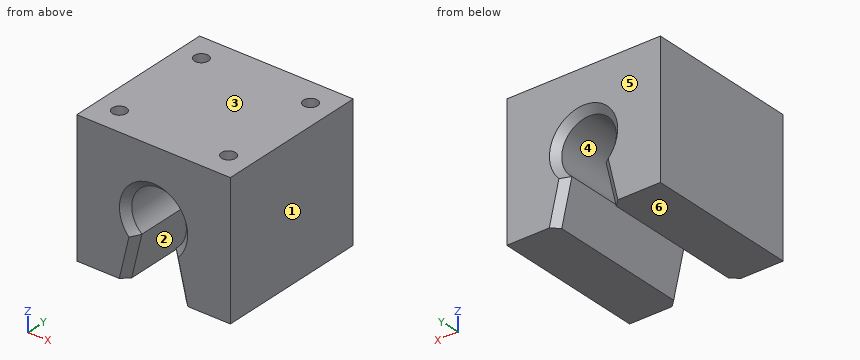
Autodesk Inventor part; units mm, degrees
ref_plane "YZ Plane" through (0, 0, 0) normal (1, 0, 0) x (0, 1, 0)
ref_plane "XZ Plane" through (0, 0, 0) normal (0, 1, 0) x (-1, 0, 0)
ref_plane "XY Plane" through (0, 0, 0) normal (0, 0, 1) x (1, 0, 0)
sketch "Skizze1" plane through (0, 0, 0) normal (0, 0, 1) x (1, 0, 0)
  line L0 (-22.5, -22.5) -> (22.5, -22.5)
  line L1 (22.5, -22.5) -> (22.5, 22.5)
  line L2 (22.5, 22.5) -> (-22.5, 22.5)
  line L3 (-22.5, 22.5) -> (-22.5, -22.5)
  line L4 (-22.5, -22.5) -> (22.5, 22.5) construction
  line L5 (22.5, -22.5) -> (-22.5, 22.5) construction
  point P0 (0, 0)
  dimension "d0" = 45
  dimension "d1" = 45
extrude "Extrusion1" add sketch "Skizze1" along normal blind 39
sketch "Skizze2" plane through (-22.5, -22.5, 0) normal (0, -1, 0) x (1, 0, 0)
  line L0 (0, 0) -> (45, 0)
  line L1 (45, 0) -> (45, 39)
  line L2 (0, 39) -> (45, 39)
  line L3 (0, 0) -> (0, 39)
  circle A0 centre (22.5, 19) radius 8
  line L4 (22.5, 0) -> (22.5, 39)
  line L5 (22.5, 19) -> (22.5, -6)
  line L6 (17.5, 12.755) -> (14.5, 0)
  line L7 (27.5, 12.755) -> (30.5, 0)
  dimension "d4" = 16
  dimension "d5" = 25
  dimension "d6" = 45
  dimension "d7" = 10
  dimension "d8" = 16
extrude "Extrusion2" cut sketch "Skizze2" against normal through all contours L6 A0 L4 L0 | L4 A0 L7 L0 | A0 L4 | L4 A0
chamfer "Fase1" distance 2 angle 45 6 edges at (0, -22.5, 27) (-6.5, -22.5, 6.3775) (6.5, -22.5, 6.3775) (0, 22.5, 27) (-6.5, 22.5, 6.3775) (6.5, 22.5, 6.3775)
ref_plane "Arbeitsebene1" through (-22.5, 0, 39) normal (0, 1, 0) x (1, 0, 0)
sketch "Skizze3" plane through (0, 0, 39) normal (0, 0, 1) x (1, 0, 0)
  line L0 (-22.5, -22.5) -> (22.5, -22.5)
  line L1 (22.5, -22.5) -> (22.5, 22.5)
  line L2 (22.5, 22.5) -> (-22.5, 22.5)
  line L3 (-22.5, 22.5) -> (-22.5, -22.5)
  line L4 (16, -15) -> (-16, -15) construction
  line L5 (-16, -15) -> (-16, 15) construction
  line L6 (-16, 15) -> (16, 15) construction
  line L7 (16, 15) -> (16, -15) construction
  line L8 (16, -15) -> (-16, 15) construction
  line L9 (-16, -15) -> (16, 15) construction
  point P0 (0, 0)
  dimension "d14" = 32
  dimension "d15" = 30
hole "Bohrung1" at (-16, -15, 39) at (16, -15, 39) at (-16, 15, 39) at (16, 15, 39) direction (0, 0, -1) diameter 4.134 depth 10 tip angle 118
properties part number "Linearwagen_20_kurz" material "Aluminium 6061"
The model under review builds one solid part; all positions refer to its coordinate system, in mm. Face numbers are marked on the shaded views. A direction names the side the tool comes from. Round coordinates to 2 decimals unless told otherwise and drop trailing zeros. Write each loop counter-clockwise with the first axis right and the second up, starting at its lowest first coordinate (ties: lowest second). Pieces come first, ordered by that corner, then holes. Notation, with made-up numbers: M 23,61 L 40,61 A23 cw 40,70 Z; hole C -5,8.25 d7. An arc over 180 degrees is marked long. Use a Markdown table: item, result. Add a question column.
Q1. The part is to be moulded in two halves that separate along Z. For the marked faces 3, 4, 5 and 6, say which applies: pulls with the +Z half, pulls with the -Z half, needs draft (parallel to the pull), parting line crosses it, or undercut.
Q2. Insertion check: pin 1 (3.5 mm diameter, centred on x = -16, y = 15, fed in from +Z). The pin has a flat end and moves straight along its axis. Give the tip position at first contact, or say it passes through.
Q3. We need section B-B, the plane y = 5. State the section outline as (x, z) points (3 decimals), plus the area to 3 significant figures.
Q4. We need section A-A, the plane z = 19. State the section outline as (x, y) points.
Q5. Machinability: for the marked faces 1 and 2, which of the approach directions +Z, -Z, +X, -X, +Y, -Y give a long, thin tool a straight path to every point of the face, cutting with its end or side? Answer none if there is none.
Q6. To check wall thickness, follow line 1 (X direction, y = 15, z = 34); line 2 (Y direction, x = -16, z = 33); line 3 (Y direction, x = -14.5, z = 30). State the ranges of each line that lie inside material, in increasing order.
Findings below:
| question | item | result |
|---|---|---|
| 1 | face 3 | pulls with the +Z half |
| 1 | face 4 | undercut |
| 1 | face 5 | needs draft |
| 1 | face 6 | pulls with the -Z half |
| 2 | pin 1 | stops at z = 28.81 |
| 3 | outline | M -22.5,0 L -8,0 L -5,12.755 A8 cw long 5,12.755 L 8,0 L 22.5,0 L 22.5,39 L -22.5,39 Z |
| 3 | area | 1,400 mm² |
| 4 | outline | M -22.5,-22.5 L -10,-22.5 L -8,-20.5 L -8,20.5 L -10,22.5 L -22.5,22.5 Z; M 8,-20.5 L 10,-22.5 L 22.5,-22.5 L 22.5,22.5 L 10,22.5 L 8,20.5 Z |
| 5 | face 1 | +Z, -Z, +X, +Y, -Y |
| 5 | face 2 | -Z, +Y, -Y |
| 6 | line 1 | x = -22.5 to -18.07, -13.93 to 13.93, 18.07 to 22.5 |
| 6 | line 2 | y = -22.5 to -17.07, -12.93 to 12.93, 17.07 to 22.5 |
| 6 | line 3 | y = -22.5 to -16.42, -13.58 to 13.58, 16.42 to 22.5 |
